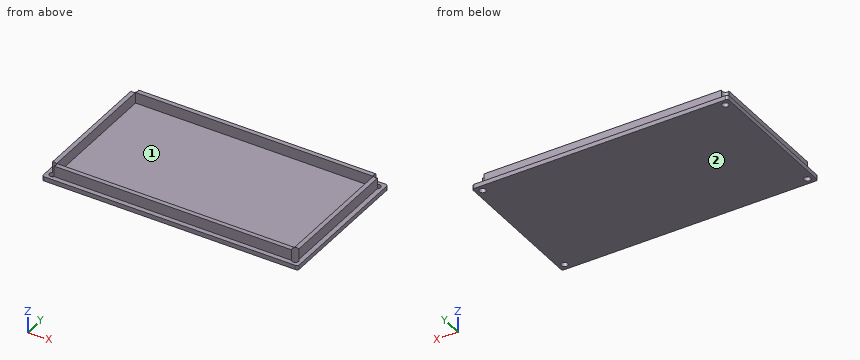
```python
from build123d import *

# Parameters (mm, degrees)
SKETCH1_W                                  = 117.9
SKETCH1_H                                  = 66.4
BOSS_EXTRUDE1_DEPTH                        = 2
SKETCH2_W                                  = 113.6
SKETCH2_H                                  = 62.1
SKETCH2_W_2                                = 109.6
SKETCH2_H_2                                = 58.1
BOSS_EXTRUDE2_DEPTH                        = 5
SKETCH3_R                                  = 1.5
CUT_EXTRUDE2_DEPTH                         = 71.854336818
MIRROR3_AT_THE_SECOND_PLANE_COPY_1_SKETC_R = 1.5
MIRROR3_AT_THE_SECOND_PLANE_COPY_1_DEPTH   = 71.854336818
FILLET1_R                                  = 1


with BuildPart() as part:
    # Sketch1 → Boss-Extrude1 (new body)
    with BuildSketch(Plane.XY):
        with Locations((3.252066252, 0)):
            Rectangle(SKETCH1_W, SKETCH1_H)
    extrude(amount=BOSS_EXTRUDE1_DEPTH)

    # Sketch2 → Boss-Extrude2 (add)
    with BuildSketch(Plane.XY.offset(2)):
        with Locations((3.252066252, 0)):
            Rectangle(SKETCH2_W, SKETCH2_H)
        with Locations((3.252066252, 0)):
            Rectangle(SKETCH2_W_2, SKETCH2_H_2, mode=Mode.SUBTRACT)
    extrude(amount=BOSS_EXTRUDE2_DEPTH)

    # Sketch3 → Cut-Extrude2 (cut, symmetric)
    with BuildSketch(Plane(origin=(0, 0, 0), x_dir=(-1, 0, 0), z_dir=(0, 0, -1))):
        with Locations(Location((-59.202066252, 30.2, 0), (0, 0, 34.518107841))):
            Circle(SKETCH3_R)
    cut_extrude2 = extrude(amount=CUT_EXTRUDE2_DEPTH, both=True, mode=Mode.SUBTRACT)

    # Mirror2: Cut-Extrude2 across plane
    add(cut_extrude2.mirror(Plane.ZX), mode=Mode.SUBTRACT)

    # Mirror3: Cut-Extrude2 across plane
    add(cut_extrude2.mirror(Plane.ZX), mode=Mode.SUBTRACT)

    # Mirror3 at the second plane: Cut-Extrude2 across plane
    add(cut_extrude2.mirror(Plane(origin=(3.252066252, 0, 0), x_dir=(0, 0, 1), z_dir=(1, 0, 0))), mode=Mode.SUBTRACT)

    # Mirror3 at the second plane copy 1 sketc → Mirror3 at the second plane copy 1 (cut, symmetric)
    with BuildSketch(Plane(origin=(6.504132503, 0, 0), x_dir=(1, 0, 0), z_dir=(0, 0, -1))):
        with Locations(Location((-59.202066252, 30.2, 0), (0, 0, 34.518107841))):
            Circle(MIRROR3_AT_THE_SECOND_PLANE_COPY_1_SKETC_R)
    extrude(amount=MIRROR3_AT_THE_SECOND_PLANE_COPY_1_DEPTH, both=True, mode=Mode.SUBTRACT)

    # Fillet1
    fillet1_edges = [part.edges().sort_by_distance(p)[0] for p in [
        (62.202066252, -33.2, 1),
        (-55.697933748, -33.2, 1),
        (-55.697933748, 33.2, 1),
        (62.202066252, 33.2, 1),
    ]]
    fillet(fillet1_edges, radius=FILLET1_R)


solid = part.part
```
Geometry check sheet. Reference: the model listing, model coordinates, mm. Face numbers are marked on the shaded views. Coordinates: 2 decimals unless noted, no trailing zeros. Order: outer loops, then holes, each group sorted by start corner. A loop starts at its lowest first (then second) coordinate and runs counter-clockwise, first axis right, second up. Notation, with made-up numbers: M 58,-2.5 L 67,-2.5 A19 ccw 67,4.5 Z; hole C 13.25,-26 d3. An arc over 180 degrees is marked long. One line per question, with ' | ' between items. Start each with the question number.
Item 1: Material ranges on L1, parallel to X at y = -27.5, z = 2.5; L2, parallel to Y at x = -49.5, z = 3.5; L3, parallel to Z at x = -32, y = -15, recorded low to high. Write a range as [from, to].
Item 2: Cross-section at B-B on z = 3.5. Enter the section's corners in (x, y), then the cut area to 3 significant figures.
Item 3: Cross-section at C-C on x = -9. Enter the section's corners in (y, z), then the cut area to 3 significant figures.
Item 4: Cross-section at A-A on y = 12.5. Enter the section's corners in (x, z), then the cut area to 3 significant figures.
Item 5: Gauge pin test, flat ends, axial feed: pin 1 (2.5 mm diameter, centred on y = -2.5, z = 5, fed in from -X); pin 2 (2 mm diameter, centred on x = -15.5, z = 5, fed in from +Y); pin 3 (4 mm diameter, centred on x = -26, z = 4.5, fed in from -Y). Record the tip position at first contact, or that the pin passes through.
Item 6: Draft check along X on the marked faces 1 and 2. Enter one of: pulls with the +X half, pulls with the -X half, needs draft (parallel to the pull), parting line crosses it, or undercut.
Findings:
1) L1: x = [-53.55, -51.55], [58.05, 60.05] | L2: y = [-31.05, -29.05], [29.05, 31.05] | L3: z = [0, 2]
2) outline: M -53.55,-28.96 A1.5 cw -51.46,-31.05 L 57.97,-31.05 A1.5 cw 60.05,-28.96 L 60.05,28.96 A1.5 cw 57.97,31.05 L -51.46,31.05 A1.5 cw -53.55,28.96 Z; hole M -51.55,-29.05 L 58.05,-29.05 L 58.05,29.05 L -51.55,29.05 Z | area: 667 mm²
3) outline: M -33.2,0 L 33.2,0 L 33.2,2 L 31.05,2 L 31.05,7 L 29.05,7 L 29.05,2 L -29.05,2 L -29.05,7 L -31.05,7 L -31.05,2 L -33.2,2 Z | area: 153 mm²
4) outline: M -55.7,0 L 62.2,0 L 62.2,2 L 60.05,2 L 60.05,7 L 58.05,7 L 58.05,2 L -51.55,2 L -51.55,7 L -53.55,7 L -53.55,2 L -55.7,2 Z | area: 256 mm²
5) pin 1: stops at x = -53.55 | pin 2: stops at y = 31.05 | pin 3: stops at y = -31.05
6) face 1: undercut | face 2: needs draft
